Read the model definition and answer for the solid it produces. Units are mm, in the model's axes. Face numbers are marked on the shaded views. Round coordinates to 2 decimals unless told otherwise and drop trailing zeros. Write each loop counter-clockwise with the first axis right and the second up, starting at its lowest first coordinate (ties: lowest second). Pieces come first, ordered by that corner, then holes. Notation, with made-up numbers: (-29.75, 46) -> (-21.75, 46) arc R25 cw to (-21.75, 69) -> close; hole circle Ø11 at (33, 75). An arc over 180 degrees is marked (long way). Return JSON: item names as keys, results as strings.
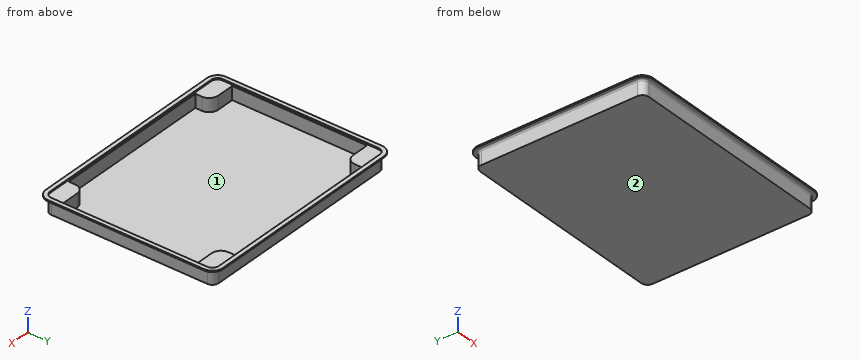
from build123d import *

# Parameters (mm, degrees)
PAD003_DEPTH    = 16
POCKET002_DEPTH = 14.5


with BuildPart() as part:
    # Sketch006 → Pad003 (new body)
    with BuildSketch(Plane.XY):
        with BuildLine():
            ThreePointArc((-110.08, 92), (-114.973179, 89.973179), (-117, 85.08))
            Line((-117, -85.08), (-117, 85.08))
            ThreePointArc((-117, -85.08), (-114.973179, -89.973179), (-110.08, -92))
            Line((110.08, -92), (-110.08, -92))
            ThreePointArc((110.08, -92), (114.973179, -89.973179), (117, -85.08))
            Line((117, 85.08), (117, -85.08))
            ThreePointArc((117, 85.08), (114.973179, 89.973179), (110.08, 92))
            Line((-110.08, 92), (110.08, 92))
        make_face()
    extrude(amount=PAD003_DEPTH)

    # Sketch007 → Pocket002 (cut)
    with BuildSketch(Plane.XY.offset(16)):
        with BuildLine():
            Line((-115.5, 73.5), (-115.5, -73.5))
            Line((-115.5, -73.5), (-96.5, -73.5))
            ThreePointArc((-86.5, -83.5), (-89.428932, -76.428932), (-96.5, -73.5))
            Line((-86.5, -90.5), (-86.5, -83.5))
            Line((86.5, -90.5), (-86.5, -90.5))
            Line((86.5, -83.5), (86.5, -90.5))
            ThreePointArc((96.5, -73.5), (89.428932, -76.428932), (86.5, -83.5))
            Line((115.5, -73.5), (96.5, -73.5))
            Line((115.5, 73.5), (115.5, -73.5))
            Line((96.5, 73.5), (115.5, 73.5))
            ThreePointArc((86.5, 83.5), (89.428932, 76.428932), (96.5, 73.5))
            Line((86.5, 90.5), (86.5, 83.5))
            Line((-86.5, 90.5), (86.5, 90.5))
            Line((-86.5, 90.5), (-86.5, 83.5))
            ThreePointArc((-96.5, 73.5), (-89.428932, 76.428932), (-86.5, 83.5))
            Line((-115.5, 73.5), (-96.5, 73.5))
        make_face()
    extrude(amount=-POCKET002_DEPTH, mode=Mode.SUBTRACT)

    # AdditivePipe001: sweep along a path in Sketch009
    with BuildLine(Plane.XY.offset(16)) as additivepipe001_path:
        ThreePointArc((-110.08, 92), (-114.973179, 89.973179), (-117, 85.08))
        Line((-117, 85.08), (-117, -85.08))
        ThreePointArc((-117, -85.08), (-114.973179, -89.973179), (-110.08, -92))
        Line((-110.08, -92), (110.08, -92))
        ThreePointArc((110.08, -92), (114.973179, -89.973179), (117, -85.08))
        Line((117, -85.08), (117, 85.08))
        ThreePointArc((117, 85.08), (114.973179, 89.973179), (110.08, 92))
        Line((110.08, 92), (-110.08, 92))
    # Sketch008 → AdditivePipe001 (sweep)
    with BuildSketch(Plane.XZ):
        with BuildLine():
            Line((117, 14.5), (117, 16))
            Line((117, 17.5), (117, 16))
            Line((121.5, 17.5), (117, 17.5))
            Line((121.5, 16), (121.5, 17.5))
            Line((118.5, 16), (121.5, 16))
            ThreePointArc((118.5, 16), (117.43934, 15.56066), (117, 14.5))
        make_face()
    sweep(path=additivepipe001_path.line)


solid = part.part
Item 1: For a pull along Y with two mould halves and no side action, classify the marked faces 1 and 2 as released by +Y, released by -Y, zero draft, split by the parting line, or undercut.
Worked answers:
{"face 1": "undercut", "face 2": "zero draft"}
Item 2: Straight lines are drawn through the part: L1, parallel to X at y = -36.5, z = 13.75; L2, parallel to Y at x = -62.5, z = 14.25; L3, parallel to X at y = 87.5, z = 15.5. For each, find the intervals that lie inside material, in ascending order. Write a range as [from, to].
Worked answers:
{"L1": "x = [-117, -115.5], [115.5, 117]", "L2": "y = [-92, -90.5], [90.5, 92]", "L3": "x = [-116.97, -86.5], [86.5, 116.97]"}
Item 3: Flat-ended cylindrical pins translate along their axes: pin 1 (6 mm diameter, centred on x = 77, z = 11.5, fed in from +Y); pin 2 (5.5 mm diameter, centred on y = 88.5, z = 7.5, fed in from +X); pin 3 (10 mm diameter, centred on x = 28, y = 8.5, fed in from +Z). Find the tip coordinate at first contact, or state that the pin passes through.
Worked answers:
{"pin 1": "stops at y = 92", "pin 2": "stops at x = 116.97", "pin 3": "stops at z = 1.5"}
Item 4: Section A-A (z = 5.5) is taken. Give the vertices of the cut face in (x, y), then the cut area to 3 significant figures.
Worked answers:
{"outline": "(-117, -85.08) arc R6.92 ccw to (-110.08, -92) -> (110.08, -92) arc R6.92 ccw to (117, -85.08) -> (117, 85.08) arc R6.92 ccw to (110.08, 92) -> (-110.08, 92) arc R6.92 ccw to (-117, 85.08) -> close; hole (-115.5, -73.5) -> (-96.5, -73.5) arc R10 cw to (-86.5, -83.5) -> (-86.5, -90.5) -> (86.5, -90.5) -> (86.5, -83.5) arc R10 cw to (96.5, -73.5) -> (115.5, -73.5) -> (115.5, 73.5) -> (96.5, 73.5) arc R10 cw to (86.5, 83.5) -> (86.5, 90.5) -> (-86.5, 90.5) -> (-86.5, 83.5) arc R10 cw to (-96.5, 73.5) -> (-115.5, 73.5) -> close", "area": "3,090 mm2"}
